from build123d import *

# Parameters (mm, degrees)
F0_W     = 110.33576
F0_H     = 54.586928
F1_DEPTH = 25
F2_T     = -2.5
F3_R     = 5.270702
F4_DEPTH = 25.001


with BuildPart() as f1:
    # F0 (on Top) → F1 (new body)
    with BuildSketch(Plane.XY):
        Rectangle(F0_W, F0_H)
    extrude(amount=F1_DEPTH)

    # F2
    f2_openings = [f1.faces().sort_by_distance(p)[0] for p in [
        (0, 0, 25),
    ]]
    offset(amount=F2_T, openings=f2_openings)

    # F3 (on Top) → F4 (cut, through all)
    with BuildSketch(Plane.XY):
        with Locations((-38.874775, 10.714518)):
            Circle(F3_R)
    extrude(amount=F4_DEPTH, mode=Mode.SUBTRACT)


solid = f1.part
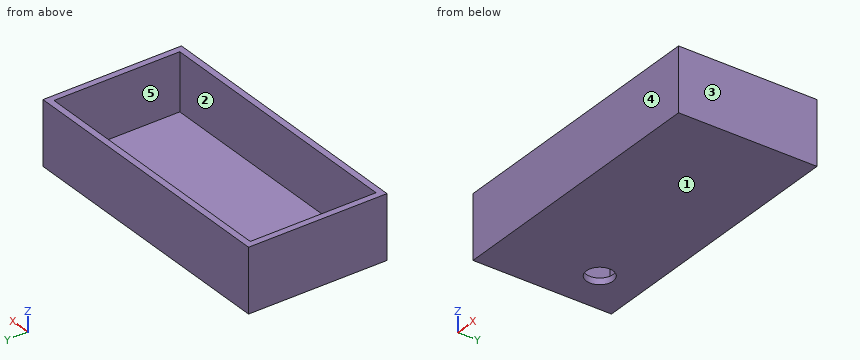
Could you check a few things on this model? Use its own coordinates, in mm. Face numbers are marked on the shaded views. A direction names the side the tool comes from. Give positions to 0.01 mm unless a question says otherwise; leave off trailing zeros. Write each loop counter-clockwise with the first axis right and the second up, starting at its lowest first coordinate (ties: lowest second). Pieces come first, ordered by that corner, then holes. Notation, with made-up numbers: (36.25, -23) -> (53.25, -23) arc R17 cw to (53.25, -16) -> close; hole circle Ø7 at (49.25, 62). An arc over 180 degrees is marked (long way). Write each question's results on one line, items separated by ' | '. Start each with the question number.
Q1. I'm going to push flat-ended pins straight in: pin 1 Ø15 at (x, y) = (-5.5, -11.5) entering from +Z; pin 2 Ø3 at (x, y) = (19.5, -19.5) entering from -Z. Where does each tip first touch, or does it pass through?
Q2. I need wall thicknesses on probe 1 along Y at (x, z) = (45, 16.5); probe 2 along X at (y, z) = (17.5, 18); probe 3 along Z at (x, y) = (-5.5, -18). Which ranges of each line are inside material? Lowest first, please.
Q3. Suppose I cut it at B-B, the plane y = -15.5. List the corners of the cut face in (x, z) for me, and give its area (3 significant figures).
Q4. Suppose I cut it at D-D, the plane x = -3. List the corners of the cut face in (y, z) for me.
Q5. We'd pull the mould along Y, two halves only. Please class the marked faces 3, 4 and 5: +Y half, -Y half, draft (parallel to the pull), parting line (faces both ways), or undercut.
Q6. Suppose I cut it at A-A, the plane z = 9. List the corners of the cut face in (x, y) for me.
Q7. Suppose I cut it at C-C, the plane x = -35. List the corners of the cut face in (y, z) for me, and give its area (3 significant figures).
Q8. Which directions (+Z, -Z, +X, -X, +Y, -Y) give clear straight access to the entire face, cutting with the end or side of a thin tool? Please do the marked faces 1 and 2.
Outcome:
1) pin 1: z = 2.5 | pin 2: z = 0
2) probe 1: -27.29 to -24.79, 24.79 to 27.29 | probe 2: -55.17 to -52.67, 52.67 to 55.17 | probe 3: 0 to 2.5
3) outline: (-55.17, 0) -> (55.17, 0) -> (55.17, 25) -> (52.67, 25) -> (52.67, 2.5) -> (-52.67, 2.5) -> (-52.67, 25) -> (-55.17, 25) -> close | area: 388 mm2
4) outline: (-27.29, 0) -> (27.29, 0) -> (27.29, 25) -> (24.79, 25) -> (24.79, 2.5) -> (-24.79, 2.5) -> (-24.79, 25) -> (-27.29, 25) -> close
5) face 3: draft | face 4: -Y half | face 5: undercut
6) outline: (-55.17, -27.29) -> (55.17, -27.29) -> (55.17, 27.29) -> (-55.17, 27.29) -> close; hole (-52.67, -24.79) -> (52.67, -24.79) -> (52.67, 24.79) -> (-52.67, 24.79) -> close
7) outline: (-27.29, 0) -> (7.14, 0) -> (7.14, 2.5) -> (-24.79, 2.5) -> (-24.79, 25) -> (-27.29, 25) -> close; (14.29, 0) -> (27.29, 0) -> (27.29, 25) -> (24.79, 25) -> (24.79, 2.5) -> (14.29, 2.5) -> close | area: 231 mm2
8) face 1: -Z, +X, -X, +Y, -Y | face 2: +Z
